Autodesk Fusion 360 part; units mm, degrees
sketch "Sketch2" plane through (0, 0, 0) normal (0, 0, 1) x (1, 0, 0)
  arc A0 (18.5, 20) -> (18, 20.5) centre (18, 20) ccw
  line L0 (18.5, 20) -> (18.5, 8.6168)
  arc A1 (18.5, 8.6168) -> (21.6842, 3.6281) centre (24, 8.6168) ccw
  arc A2 (20, -4) -> (21.6842, 3.6281) centre (20, 0) ccw
  line L1 (20, -4) -> (0, -4)
  arc A3 (-1.6842, 3.6281) -> (0, -4) centre (0, 0) ccw
  arc A4 (-1.6842, 3.6281) -> (1.5, 8.6168) centre (-4, 8.6168) ccw
  line L2 (1.5, 8.6168) -> (1.5, 20)
  arc A5 (2, 20.5) -> (1.5, 20) centre (2, 20) ccw
  line L3 (2, 20.5) -> (18, 20.5)
  circle A6 centre (20, 0) radius 1.1
  circle A7 centre (0, 0) radius 1.1
  line L4 (24, 9) -> (-4, 9)
  line L5 (-4, 0) -> (-4, 9)
  line L6 (24, 0) -> (24, 9)
  line L7 (1.5, 9) -> (1.5, 5)
  line L8 (1.5, 5) -> (18.5, 5)
  line L9 (18.5, 5) -> (18.5, 9)
  line L10 (10, -4) -> (10, 20.5) construction
  point P0 (4, 2.5)
  point P1 (16, 2.5)
  dimension "d2" = 9
  dimension "d6" = 4
  dimension "d20" = 12
  dimension "d21" = 2.5
ref_plane "WorkPlane1" through (0, 9, 0) normal (0, 1, 0) x (0, 0, 1)
sketch "Sketch3" plane through (0, 9, 0) normal (0, 1, 0) x (1, 0, 0)
  circle A0 centre (4, -13.5) radius 0.625
  circle A1 centre (4, -13.5) radius 0.625
  circle A2 centre (16, -13.5) radius 0.625
  circle A3 centre (16, -13.5) radius 0.625
  circle A4 centre (16, -1.5) radius 0.625
  circle A5 centre (16, -1.5) radius 0.625
  circle A6 centre (4, -1.5) radius 0.625
  circle A7 centre (4, -1.5) radius 0.625
  dimension "d4" = 12
  dimension "d5" = 12
extrude "Extrude1" add sketch "Sketch2" along normal blind 2.5 and the other way blind 0.5 contours L0 A1 A2 L4 L6 L9 | L0 L2 L4 L7 L8 L9 | A1 A2 L1 A3 A4 L7 L8 L9 | A3 A4 L2 L4 L5 L7
extrude "Extrude2" add sketch "Sketch2" along normal blind 16 contours L0 L2 L4 L7 L8 L9
hole "Hole1" at (4, 9, 13.5) at (16, 9, 13.5) at (16, 9, 1.5) at (4, 9, 1.5) direction (0, -1, 0) diameter 1.271 depth 6.5 tip angle 118
fillet "Fillet1" radius 4 2 edges at (24, 9, 1) (-4, 9, 1)
fillet "Fillet1" radius 0.5 4 edges at (18.5, 9, 9.25) (1.5, 9, 9.25) (18.5, 5, 9.25) (1.5, 5, 9.25)
hole "Hole2" at (16, 2.5, 0) at (4, 2.5, 0) direction (0, 0, -1) diameter 2.2 depth 11 tip angle 118
hole "Hole3" at (16, 2.5, 0) at (4, 2.5, 0) direction (0, 0, 1) diameter 2.2 depth 11 tip angle 118
Geometry check sheet. Reference: the model listing, model coordinates, mm. A direction names the side the tool comes from. Round coordinates to 2 decimals unless told otherwise and drop trailing zeros. Order: outer loops, then holes, each group sorted by start corner. A loop starts at its lowest first (then second) coordinate and runs counter-clockwise, first axis right, second up. Notation, with made-up numbers: M -34,68 L 2,68 A7 ccw 2,72 Z; hole C 77,70.25 d10. An arc over 180 degrees is marked long. Answer as CSV lines item,"result".
1) Sectioned sample at D-D on x = 7.25. Record the cut outline in (y, z).
Entries:
outline,"M -4,-0.5 L 9,-0.5 L 9,16 L 5,16 L 5,2.5 L -4,2.5 Z"
2) Sectioned sample at C-C on y = 4.5. Record the cut outline in (x, z).
Entries:
outline,"M -4,-0.5 L 24,-0.5 L 24,2.5 L -4,2.5 Z; hole C 4,1.5 d1.27; hole C 16,1.5 d1.27"
3) Mould release check, pull along Z, two halves, no side actions. Record for faces 5 (the face through (-4, 2, 1)), 6 (the face through (16.62, 6.16, 1.36)), 7 (the face through (10, 1, 2.5)): +Z half, -Z half, draft (parallel to the pull), parting line (faces both ways), or undercut.
Entries:
face 5,"draft"
face 6,"undercut"
face 7,"+Z half"
4) Gauge pin test, flat ends, axial feed: pin 1 Ø3 at (x, z) = (4.5, 10) entering from -Y; pin 2 Ø0.9 at (y, z) = (7, 11.5) entering from +X; pin 3 Ø1 at (y, z) = (7, 2) entering from +X; pin 4 Ø1.7 at (x, z) = (16, 1.5) entering from +Y. Record the tip position at first contact, or that the pin passes through.
Entries:
pin 1,"y = 5"
pin 2,"x = 18.5"
pin 3,"x = 23.71"
pin 4,"y = 9"
5) Sectioned sample at B-B on z = 13.5. Record the cut outline in (x, y), and give its area (3 significant figures).
Entries:
outline,"M 1.5,5.5 A0.5 ccw 2,5 L 3.36,5 L 3.36,9 L 2,9 A0.5 ccw 1.5,8.5 Z; M 4.64,5 L 15.36,5 L 15.36,9 L 4.64,9 Z; M 16.64,5 L 18,5 A0.5 ccw 18.5,5.5 L 18.5,8.5 A0.5 ccw 18,9 L 16.64,9 Z"
area,"57.6 mm2"
6) Sectioned sample at A-A on y = 2.5. Record the cut outline in (x, z).
Entries:
outline,"M -4,-0.5 L 2.9,-0.5 L 2.9,2.5 L -4,2.5 Z; M 5.1,-0.5 L 14.9,-0.5 L 14.9,2.5 L 5.1,2.5 Z; M 17.1,-0.5 L 24,-0.5 L 24,2.5 L 17.1,2.5 Z"
7) Tool access check on faces 1 (the face through (1.05, -0.33, 0.98)), 2 (the face through (10, 5, 9)), 3 (the face through (1.5, 7, 9)), 4 (the face through (3.972, 6.16, 0.865)). Record the directions out of +Z, -Z, +X, -X, +Y, -Y that give a thin tool (end or side, any length) a straight path to the whole face; none if there is none.
Entries:
face 1,"+Z, -Z"
face 2,"+Z, +X, -X, -Y"
face 3,"+Z, -X, +Y, -Y"
face 4,"+Y"
8) Thickness scan on probe 1 along X at (y, z) = (5.2, 1.5) (1 decimal); probe 2 along Z at (x, y) = (16, 5.6); probe 3 along Y at (x, z) = (16, 0.45). Record the ranges inside material, lowest first. Write a range as [from, to].
Entries:
probe 1,"[-4, 3.4], [4.6, 15.4], [16.6, 24]"
probe 2,"[-0.5, 0.86], [2.14, 12.86], [14.14, 16]"
probe 3,"[-4, 1.4], [3.6, 9]"
